The model under review builds one solid part; all positions refer to its coordinate system, in mm. Face numbers are marked on the shaded views. Round coordinates to 2 decimals unless told otherwise and drop trailing zeros. Write each loop counter-clockwise with the first axis right and the second up, starting at its lowest first coordinate (ties: lowest second). Pieces come first, ordered by that corner, then holes. Notation, with made-up numbers: (30.25, 9) -> (66.25, 9) arc R26 ccw to (66.25, 26) -> close; hole circle Ø6 at (85.5, 3.5). An arc over 180 degrees is marked (long way). Answer as a JSON object with one key per item and string values. Group by question number.
1) We need section A-A, the plane y = 14.85. Write out the cut boundary in (x, z).
2) To check wall thickness, follow probe 1 along Y at (x, z) = (-15, 32); probe 2 along X at (y, z) = (14, 35); probe 3 along X at (y, z) = (23.5, 31.5). State the ranges of each line that lie inside material, in increasing order. Write a range as [from, to].
3) We need section C-C, the plane z = 13. Write out the cut boundary in (x, y), then the cut area to 3 significant figures.
4) We need section B-B, the plane x = -15.3. Write out the cut boundary in (y, z).
5) Mouldability with a two-part tool opening along X and no side actions: class the marked faces 1, 2 and 3 as pulls with the +X half, pulls with the -X half, needs draft (parallel to the pull), parting line crosses it, or undercut.
from build123d import *

# Parameters (mm, degrees)
F0_W     = 80
F0_H     = 80
F1_DEPTH = 80
F2_R     = 15
F3_DEPTH = 80.001
F4_R     = 5
F5_R     = 5


with BuildPart() as f1:
    # F0 (on Top) → F1 (new body)
    with BuildSketch(Plane.XY):
        with Locations((-14.930487, 14.1732)):
            Rectangle(F0_W, F0_H)
    extrude(amount=F1_DEPTH)

    # F2 (on face) → F3 (cut, through all)
    with BuildSketch(Plane.XY.offset(80)):
        with Locations((-15.300001, 14.85)):
            Circle(F2_R)
    extrude(amount=-F3_DEPTH, mode=Mode.SUBTRACT)

    # F4
    f4_edges = [f1.edges().sort_by_distance(p)[0] for p in [
        (-14.930487, -25.8268, 0),
        (-54.930487, 14.1732, 0),
        (25.069513, 14.1732, 0),
        (-14.930487, 54.1732, 0),
    ]]
    fillet(f4_edges, radius=F4_R)

    # F5
    f5_edges = [f1.edges().sort_by_distance(p)[0] for p in [
        (-14.930487, 54.1732, 80),
        (-54.930487, 14.1732, 80),
        (-14.930487, -25.8268, 80),
        (25.069513, 14.1732, 80),
    ]]
    fillet(f5_edges, radius=F5_R)


solid = f1.part
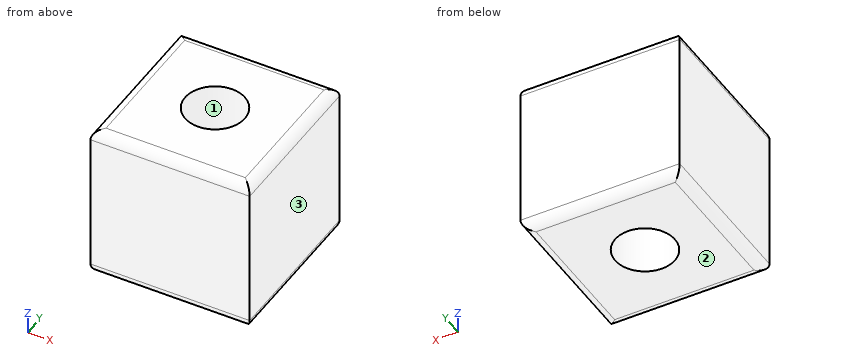
Here are the results:
{
 "1": {"outline": "(-54.93, 5) arc R5 ccw to (-49.93, 0) -> (-30.3, 0) -> (-30.3, 80) -> (-49.93, 80) arc R5 ccw to (-54.93, 75) -> close; (-0.3, 0) -> (20.07, 0) arc R5 ccw to (25.07, 5) -> (25.07, 75) arc R5 ccw to (20.07, 80) -> (-0.3, 80) -> close"},
 "2": {"probe 1": "y = [-25.83, -0.15], [29.85, 54.17]", "probe 2": "x = [-54.93, -30.28], [-0.32, 25.07]", "probe 3": "x = [-54.93, -27.55], [-3.05, 25.07]"},
 "3": {"outline": "(-54.93, -25.83) -> (25.07, -25.83) -> (25.07, 54.17) -> (-54.93, 54.17) -> close; hole circle Ø30 at (-15.3, 14.85)", "area": "5,690 mm^2"},
 "4": {"outline": "(-25.83, 5) arc R5 ccw to (-20.83, 0) -> (-0.15, 0) -> (-0.15, 80) -> (-20.83, 80) arc R5 ccw to (-25.83, 75) -> close; (29.85, 0) -> (49.17, 0) arc R5 ccw to (54.17, 5) -> (54.17, 75) arc R5 ccw to (49.17, 80) -> (29.85, 80) -> close"},
 "5": {"face 1": "undercut", "face 2": "needs draft", "face 3": "pulls with the +X half"}
}
